Here's how the part is built. I have some questions about the finished solid (model axes, mm). A direction names the side the tool comes from. Give positions to 0.01 mm unless a question says otherwise; leave off trailing zeros. Loops run counter-clockwise (first coordinate to the right, second up) from the corner with the lowest first, then second, coordinate; pieces in that order, holes last. Notation, with made-up numbers: M -34,1 L -20,1 A23 cw -20,9 Z; hole C 47,41 d5. An arc over 180 degrees is marked long. Answer as CSV lines item,"result". Start each with the question number.
Item 1: If we mould it in two halves opening along Y, with no side actions, what happens to faces 5 (the flat face through (8, 0, -39)), 6 (the flat face through (10.76, 15.42, 2.46)), 7 (the flat face through (6, 15, 5))? For each: released by +Y, released by -Y, zero draft, split by the parting line, or undercut.
Item 2: If I drill on line 1 along Y through (x, z) = (13.25, -37); line 2 along Y through (x, z) = (10.5, -33.5); line 3 along Z through (x, y) = (5.5, 34.5), over which ranges is the centre line in solid material (lowest first)? Write a range as from..to.
Item 3: I want a section at B-B on y = 50. List the corners of the cut face in (x, z) for me.
Item 4: I want a section at A-A on z = -36.5. List the corners of the cut face in (x, y) for me, plus the area to 3 significant figures.
Item 5: For faces 1 (the flat face through (8, 6, -35)), 2 (the flat face through (5.08, 15.36, 2.46)), 3 (the flat face through (1.972, 51.563, -1.479)), 4 (the flat face through (4, 52, 2)), which set-ups out of +Z, -Z, +X, -X, +Y, -Y let a thin tool reach every point of the face, with its end or its side?
Item 6: I want a section at D-D on x = 10.75. List the corners of the cut face in (y, z) for me, plus the area to 3 significant figures.
Item 7: Will these pins go through, and if not, where does the flat tip stop? P1, Ø1, axis at y = 14.5, z = -37, coming from the -X side; P2, Ø3.5, axis at y = 37.5, z = -2, coming from the -X side; P3, Ø0.7, axis at x = 10, y = 3, coming from the +Z side; P4, Ø3, axis at x = 11.5, z = -27, coming from the -Y side.
Item 8: I want a section at C-C on z = -1.5. List the corners of the cut face in (x, y) for me, plus the area to 3 significant figures.
Autodesk Inventor part; units mm, degrees
ref_plane "YZ Plane" through (0, 0, 0) normal (1, 0, 0) x (0, 1, 0)
ref_plane "XZ Plane" through (0, 0, 0) normal (0, 1, 0) x (-1, 0, 0)
ref_plane "XY Plane" through (0, 0, 0) normal (0, 0, 1) x (1, 0, 0)
sketch "Sketch1" plane through (0, 0, 0) normal (0, 0, 1) x (1, 0, 0)
  line L0 (0, 0) -> (0, 20)
  line L1 (0, 20) -> (16, 20)
  line L2 (16, 20) -> (16, 0)
  line L3 (16, 0) -> (0, 0)
  line L4 (8, 28) -> (0, 20)
  line L5 (8, 28) -> (16, 20)
  line L6 (0, 0) -> (0, 5)
  line L7 (0, 0) -> (0, 1.5)
  line L8 (0, 5) -> (0, 3.5)
  line L9 (1.5, 3.5) -> (1.5, 1.5)
  line L10 (1.5, 3.5) -> (14.5, 3.5)
  line L11 (14.5, 3.5) -> (14.5, 1.5)
  line L12 (14.5, 1.5) -> (1.5, 1.5)
  line L13 (14.5, 18.5) -> (15.1649, 19.1649)
  line L14 (15.1649, 19.1649) -> (0.8351, 19.1649)
  line L15 (0.8351, 19.1649) -> (1.5, 18.5)
  line L16 (1.5, 18.5) -> (14.5, 18.5)
  line L17 (12, 17.6183) -> (4, 17.6183)
  line L18 (4, 17.6183) -> (8.0319, 13.6184)
  line L19 (8.0319, 13.6184) -> (12, 17.6183)
  line L20 (12.4747, 17.1474) -> (13.3985, 16.231)
  line L21 (13.3985, 16.231) -> (10.016, 12.8213)
  line L22 (10.016, 12.8213) -> (9.0922, 13.7377)
  line L23 (9.0922, 13.7377) -> (12.4747, 17.1474)
  line L24 (6.8378, 13.6184) -> (3.2805, 17.1474)
  line L25 (3.2805, 17.1474) -> (2.3714, 16.231)
  line L26 (2.3714, 16.231) -> (5.9286, 12.702)
  line L27 (5.9286, 12.702) -> (6.8378, 13.6184)
  dimension "d0" = 20
  dimension "d1" = 16
  dimension "d3" = 5
  dimension "d7" = 1.5
  dimension "d9" = 13
extrude "Extrusion1" add sketch "Sketch1" along normal blind 5
extrude "Extrusion2" add sketch "Sketch1" along normal blind 4 contours L10 L11 L12 L9
sketch "Sketch2" plane through (0, 0, 0) normal (0, 0, -1) x (-1, 0, 0)
  line L0 (-16, 20) -> (-8, 28)
  line L1 (-16, 20) -> (0, 20)
  line L2 (0, 20) -> (-8, 28)
  line L3 (-16, 20) -> (-16, 56)
  line L4 (-16, 20) -> (20, 20) construction
  line L5 (-16, 56) -> (0, 56)
  line L6 (0, 56) -> (0, 20)
  line L7 (-16, 56) -> (-8, 48)
  line L8 (-16, 56) -> (-4.6863, 56) construction
  line L9 (-8, 48) -> (0, 56)
  point P0 (0, 0)
  dimension "d12" = 36
  dimension "d13" = 90
  dimension "d14" = 45
extrude "Extrusion3" add sketch "Sketch2" against normal blind 5 contours L5 L9 L7
sketch "Sketch3" plane through (0, 0, 0) normal (0, 0, -1) x (-1, 0, 0)
  line L0 (0, 56) -> (-8, 48)
  line L1 (-16, 0) -> (-16, 20)
  line L2 (0, 56) -> (-16, 56)
  line L3 (-16, 56) -> (-16, 0)
  line L4 (-16, 0) -> (0, 0)
  line L5 (0, 0) -> (0, 56)
  line L6 (-16, 20) -> (-8, 28)
  line L7 (-16, 20) -> (0, 20)
  line L8 (-8, 28) -> (0, 20)
  line L9 (-8, 28) -> (-8, 48)
  line L10 (-16, 56) -> (-8, 38)
  line L11 (0, 56) -> (-8, 38)
  line L12 (-8, 38) -> (0, 20)
  line L13 (-8, 38) -> (-16, 20)
  line L14 (-12, 47) -> (-12, 29)
  line L15 (-4, 47) -> (-4, 29)
  point P0 (0, 0)
extrude "Extrusion4" add sketch "Sketch3" along normal blind 3 contours L11 L9 L0 | L0 L9 L10 L2 | L5 L4 L1 L7 | L7 L6 L8 | L8 L9 L12 | L15 L12 L11 | L13 L14 L10 | L9 L6 L13
sketch "Sketch4" plane through (0, 0, 5) normal (0, 0, 1) x (1, 0, 0)
  line L0 (0, 0) -> (0, 20)
  line L1 (16, 20) -> (16, 0)
  line L2 (0, 0) -> (16, 0)
  line L3 (16, 0) -> (16, 10)
  line L4 (16, 10) -> (0, 10)
  line L5 (0, 10) -> (0, 0)
extrude "Extrusion5" cut sketch "Sketch4" against normal blind 10
sketch "Sketch5" plane through (0, 0, -3) normal (0, 0, -1) x (-1, 0, 0)
  line L0 (0, 10) -> (-16, 10)
  line L1 (0, 10) -> (0, 20)
  line L2 (-16, 10) -> (0, 10)
  line L3 (0, 10) -> (0, 15)
  line L4 (0, 15) -> (-16, 15)
  line L5 (-16, 15) -> (-16, 10)
  point P0 (0, 0)
  dimension "d21" = 5
extrude "Extrusion6" add sketch "Sketch5" along normal blind 40
sketch "Sketch6" plane through (0, 10, 5) normal (0, -1, 0) x (1, 0, 0)
  line L0 (16, -48) -> (0, -48)
  line L1 (16, 0) -> (16, -48)
  line L2 (0, -48) -> (16, -48)
  line L3 (16, -48) -> (16, -40)
  line L4 (16, -40) -> (0, -40)
  line L5 (0, -40) -> (0, -48)
  point P0 (0, -5)
  dimension "d24" = 8
extrude "Extrusion7" add sketch "Sketch6" along normal blind 10
sketch "Sketch7" plane through (0, 10, -35) normal (0, 0, 1) x (1, 0, 0)
  line L0 (0, -10) -> (16, -10)
  line L1 (16, -10) -> (16, -5)
  line L2 (16, -5) -> (0, -5)
  line L3 (0, -5) -> (0, -10)
  line L4 (0, -10) -> (1.5, -10)
  line L5 (1.5, -10) -> (1.5, -8.5)
  line L6 (1.5, -8.5) -> (0, -8.5)
  line L7 (0, -8.5) -> (0, -10)
  line L8 (1.5, -8.5) -> (14.5, -8.5)
  line L9 (14.5, -8.5) -> (14.5, -6.3)
  line L10 (14.5, -6.3) -> (1.5, -6.3)
  line L11 (1.5, -6.3) -> (1.5, -8.5)
  dimension "d27" = 16
  dimension "d28" = 5
  dimension "d29" = 1.5
  dimension "d30" = 1.5
  dimension "d31" = 13
  dimension "d32" = 2.2
extrude "Extrusion8" cut sketch "Sketch7" against normal blind 3 contours L11 L10 L9 L8
properties part number "Connecting pt.2"
Result:
1,face 5,"released by -Y"
1,face 6,"undercut"
1,face 7,"zero draft"
2,line 1,"0..1.5, 3.7..15"
2,line 2,"10..15"
2,line 3,"-3..0"
3,outline,"M 2.67,-3 L 13.33,-3 L 13.33,0 L 10,0 L 10,5 L 6,5 L 6,0 L 2.67,0 Z"
4,outline,"M 0,0 L 16,0 L 16,15 L 0,15 Z; hole M 1.5,1.5 L 14.5,1.5 L 14.5,3.7 L 1.5,3.7 Z"
4,area,"211 mm^2"
5,face 1,"+Z, +X, -X, -Y"
5,face 2,"+Z"
5,face 3,"+Z, -Z, -X"
5,face 4,"+Z, -X"
6,outline,"M 0,-43 L 15,-43 L 15,-3 L 56,-3 L 56,5 L 50.75,5 L 50.75,0 L 25.25,0 L 25.25,5 L 19.16,5 L 19.16,0 L 18.5,0 L 18.5,5 L 17.62,5 L 17.62,0 L 16.36,0 L 16.36,5 L 15.41,5 L 15.41,0 L 13.56,0 L 13.56,5 L 10,5 L 10,-35 L 3.7,-35 L 3.7,-38 L 1.5,-38 L 1.5,-35 L 0,-35 Z"
6,area,"495 mm^2"
7,P1,"x = 0"
7,P2,"x = 4"
7,P3,"z = -38"
7,P4,"y = 10"
8,outline,"M 0,10 L 16,10 L 16,20 L 12,29 L 12,47 L 16,56 L 0,56 L 4,47 L 4,29 L 0,20 Z"
8,area,"520 mm^2"
